from build123d import *

# Parameters (mm, degrees)
BOSS_EXTRUDE1_DEPTH        = 44
F_21_0_21_DIAMETER_HOLE1_D = 21
F_26_0_26_DIAMETER_HOLE1_D = 26
BOSS_EXTRUDE2_START        = -1.5
SKETCH9_R                  = 10.5
SKETCH9_R_2                = 8.75
BOSS_EXTRUDE2_DEPTH        = 1.5
BOSS_EXTRUDE3_START        = 88
SKETCH9_2_R                = 10.5
SKETCH9_2_R_2              = 8.75
BOSS_EXTRUDE3_DEPTH        = 1.5
SKETCH16_R                 = 13
SKETCH16_R_2               = 11.25
BOSS_EXTRUDE4_DEPTH        = 1.5
SKETCH17_W                 = 18.25
SKETCH17_H                 = 1.5
CUT_EXTRUDE1_DEPTH         = 80.504716841
CUT_EXTRUDE3_DEPTH         = 121.137421314
FILLET3_R                  = 5


with BuildPart() as part:
    # Sketch1 → Boss-Extrude1 (new body)
    with BuildSketch(Plane.XY):
        Polygon((44, 0), (-44, 0), (-44, -41), (-52, -41), (-52, 8), (52, 8), (52, -41), (44, -41), align=None)
    extrude(amount=BOSS_EXTRUDE1_DEPTH)

    # Ø21.0 (21) Diameter Hole1 (through all)
    with Locations(Plane.ZY.offset(52)):
        with Locations((22, -27)):
            Hole(F_21_0_21_DIAMETER_HOLE1_D / 2)

    # Ø26.0 (26) Diameter Hole1 (through all)
    with Locations(Plane(origin=(0, 8, 0), x_dir=(1, 0, 0), z_dir=(0, 1, 0))):
        with Locations((0, -22)):
            Hole(F_26_0_26_DIAMETER_HOLE1_D / 2)

    # Sketch9 → Boss-Extrude2 (add)
    with BuildSketch(Plane.ZY.offset(-44).offset(BOSS_EXTRUDE2_START)):
        with Locations((22, -27)):
            Circle(SKETCH9_R)
        with Locations((22, -27)):
            Circle(SKETCH9_R_2, mode=Mode.SUBTRACT)
    extrude(amount=BOSS_EXTRUDE2_DEPTH)

    # Sketch9<2> → Boss-Extrude3 (add)
    with BuildSketch(Plane.ZY.offset(-44).offset(BOSS_EXTRUDE3_START)):
        with Locations((22, -27)):
            Circle(SKETCH9_2_R)
        with Locations((22, -27)):
            Circle(SKETCH9_2_R_2, mode=Mode.SUBTRACT)
    extrude(amount=BOSS_EXTRUDE3_DEPTH)

    # Sketch16 → Boss-Extrude4 (add)
    with BuildSketch(Plane(origin=(0, 0, 0), x_dir=(1, 0, 0), z_dir=(0, 1, 0))):
        with Locations(Location((0, -22, 0), (0, 0, 270))):
            Circle(SKETCH16_R)
        with Locations(Location((0, -22, 0), (0, 0, 270))):
            Circle(SKETCH16_R_2, mode=Mode.SUBTRACT)
    extrude(amount=BOSS_EXTRUDE4_DEPTH)

    # Sketch17 → Cut-Extrude1 (cut, through all)
    with BuildSketch(Plane.XY.offset(44)):
        with Locations((0, 0.75)):
            Rectangle(SKETCH17_W, SKETCH17_H)
    extrude(amount=-CUT_EXTRUDE1_DEPTH, mode=Mode.SUBTRACT)

    # Sketch19 → Cut-Extrude3 (cut, through all)
    with BuildSketch(Plane.ZY.offset(52)):
        with BuildLine():
            ThreePointArc((0, -25), (2.087839834, -24.722753708), (4.030968204, -23.910231207))
            Line((4.030968204, -23.910231207), (0, -17))
            Line((0, -17), (0, -25))
        make_face()
        with BuildLine():
            Line((0, -17), (4.030968204, -23.910231207))
            ThreePointArc((4.030968204, -23.910231207), (6.937137221, -20.984485812), (8, -17))
            ThreePointArc((8, -17), (5.656854249, -11.343145751), (0, -9))
            Line((0, -9), (0, -17))
        make_face()
        with BuildLine():
            Line((14, -41), (8, -30.714285714))
            Line((8, -30.714285714), (4.030968204, -23.910231207))
            ThreePointArc((4.030968204, -23.910231207), (2.087839834, -24.722753708), (0, -25))
            Line((0, -25), (0, -41))
            Line((0, -41), (14, -41))
        make_face()
        with BuildLine():
            Line((4.030968204, -23.910231207), (8, -30.714285714))
            Line((8, -30.714285714), (8, -17))
            ThreePointArc((8, -17), (6.937137221, -20.984485812), (4.030968204, -23.910231207))
        make_face()
        with BuildLine():
            Line((36, -17), (36, -30.714285714))
            Line((36, -30.714285714), (39.969031796, -23.910231207))
            ThreePointArc((39.969031796, -23.910231207), (37.062862779, -20.984485812), (36, -17))
        make_face()
        with BuildLine():
            ThreePointArc((39.969031796, -23.910231207), (41.912160166, -24.722753708), (44, -25))
            Line((44, -25), (44, -17))
            Line((44, -17), (39.969031796, -23.910231207))
        make_face()
        with BuildLine():
            ThreePointArc((44, -9), (38.343145751, -11.343145751), (36, -17))
            ThreePointArc((36, -17), (37.062862779, -20.984485812), (39.969031796, -23.910231207))
            Line((39.969031796, -23.910231207), (44, -17))
            Line((44, -17), (44, -9))
        make_face()
        with BuildLine():
            Line((36, -30.714285714), (30, -41))
            Line((30, -41), (44, -41))
            Line((44, -41), (44, -25))
            ThreePointArc((44, -25), (41.912160166, -24.722753708), (39.969031796, -23.910231207))
            Line((39.969031796, -23.910231207), (36, -30.714285714))
        make_face()
    extrude(amount=-CUT_EXTRUDE3_DEPTH, mode=Mode.SUBTRACT)

    # Fillet3
    fillet3_edges = [part.edges().sort_by_distance(p)[0] for p in [
        (48, -9, 0),
        (-48, -9, 0),
        (-48, -9, 44),
        (48, -9, 44),
        (-48, -30.714285714, 36),
        (48, -30.714285714, 36),
        (-48, -41, 30),
        (48, -41, 30),
        (-48, -30.714285714, 8),
        (48, -30.714285714, 8),
        (-48, -41, 14),
        (48, -41, 14),
    ]]
    fillet(fillet3_edges, radius=FILLET3_R)


solid = part.part
Geometry check sheet. Reference: the model listing, model coordinates, mm. A direction names the side the tool comes from. Give positions to 0.01 mm unless a question says otherwise; leave off trailing zeros. Order: outer loops, then holes, each group sorted by start corner. A loop starts at its lowest first (then second) coordinate and runs counter-clockwise, first axis right, second up.
1. Scan lines: line 1 (Z direction, x = 0, y = 4.5); line 2 (Y direction, x = -49.75, z = 22); line 3 (Y direction, x = 44.5, z = 22). Record each from-to range of solid material in increasing order.
Completed:
line 1: z = 0 to 9, 35 to 44
line 2: y = -41 to -37.5, -16.5 to 8
line 3: y = -41 to -35.75, -18.25 to 8
2. Sectioned sample at A-A (z = 22). State how many separate pieces and enclosed holes the cut face has, then the cut area to 3 significant figures.
Completed:
separate pieces: 4
enclosed holes: 0
area: 960 mm2
3. Draft check along X on faces 5 (the face through (44, -16, 22)), 6 (the face through (45.5, -19, 18)), 7 (the face through (48.8, -16.59, 23.37)). Enter one of: pulls with the +X half, pulls with the -X half, needs draft (parallel to the pull), parting line crosses it, or undercut.
Completed:
face 5: undercut
face 6: pulls with the +X half
face 7: needs draft
4. Access from +Z, -Z, +X, -X, +Y, -Y to the whole of each face (thin tool, end or side, straight path). Record for faces 1 (the face through (27, 0, 22)), 2 (the face through (-48, -23, 36)), 3 (the face through (-48.7, -16.59, 23.37)), 4 (the face through (-12.3, 8, 16.8)).
Completed:
face 1: +Z, -Z, -Y
face 2: +Z, +X, -X, -Y
face 3: -X
face 4: +Z, -Z, +X, -X, +Y
5. Sectioned sample at C-C (y = -34). Record the boundary of the cut face in (x, z).
Completed:
outline: (-52, 9.92) - (-44, 9.92) - (-44, 16.75) - (-45.5, 16.75) - (-45.5, 14.17) - (-52, 14.17) - close; (-52, 29.83) - (-45.5, 29.83) - (-45.5, 27.25) - (-44, 27.25) - (-44, 34.08) - (-52, 34.08) - close; (44, 9.92) - (52, 9.92) - (52, 14.17) - (45.5, 14.17) - (45.5, 16.75) - (44, 16.75) - close; (44, 27.25) - (45.5, 27.25) - (45.5, 29.83) - (52, 29.83) - (52, 34.08) - (44, 34.08) - close
6. Depth check by flat-ended pin: pin 1 (4 mm diameter, centred on y = -34, z = 29, fed in from +X); pin 2 (1.5 mm diameter, centred on x = 9, z = 31, fed in from -Y); pin 3 (4 mm diameter, centred on x = -46.5, y = -25.5, fed in from -Z); pin 4 (15.5 mm diameter, centred on x = 0, z = 22, fed in from +Y). Enter the tip coordinate at first touch or a pass-through.
Completed:
pin 1: stops at x = 52
pin 2: stops at y = 0
pin 3: stops at z = 8
pin 4: passes through
7. Sectioned sample at D-D (y = -27). Record the boundary of the cut face in (x, z), then the cut area to 4 significant figures.
Completed:
outline: (-52, 8) - (-44, 8) - (-44, 13.25) - (-45.5, 13.25) - (-45.5, 11.5) - (-52, 11.5) - close; (-52, 32.5) - (-45.5, 32.5) - (-45.5, 30.75) - (-44, 30.75) - (-44, 36) - (-52, 36) - close; (44, 8) - (52, 8) - (52, 11.5) - (45.5, 11.5) - (45.5, 13.25) - (44, 13.25) - close; (44, 30.75) - (45.5, 30.75) - (45.5, 32.5) - (52, 32.5) - (52, 36) - (44, 36) - close
area: 122.5 mm2
8. Sectioned sample at B-B (x = 0). Record the boundary of the cut face in (y, z).
Completed:
outline: (1.5, 0) - (8, 0) - (8, 9) - (1.5, 9) - close; (1.5, 35) - (8, 35) - (8, 44) - (1.5, 44) - close
